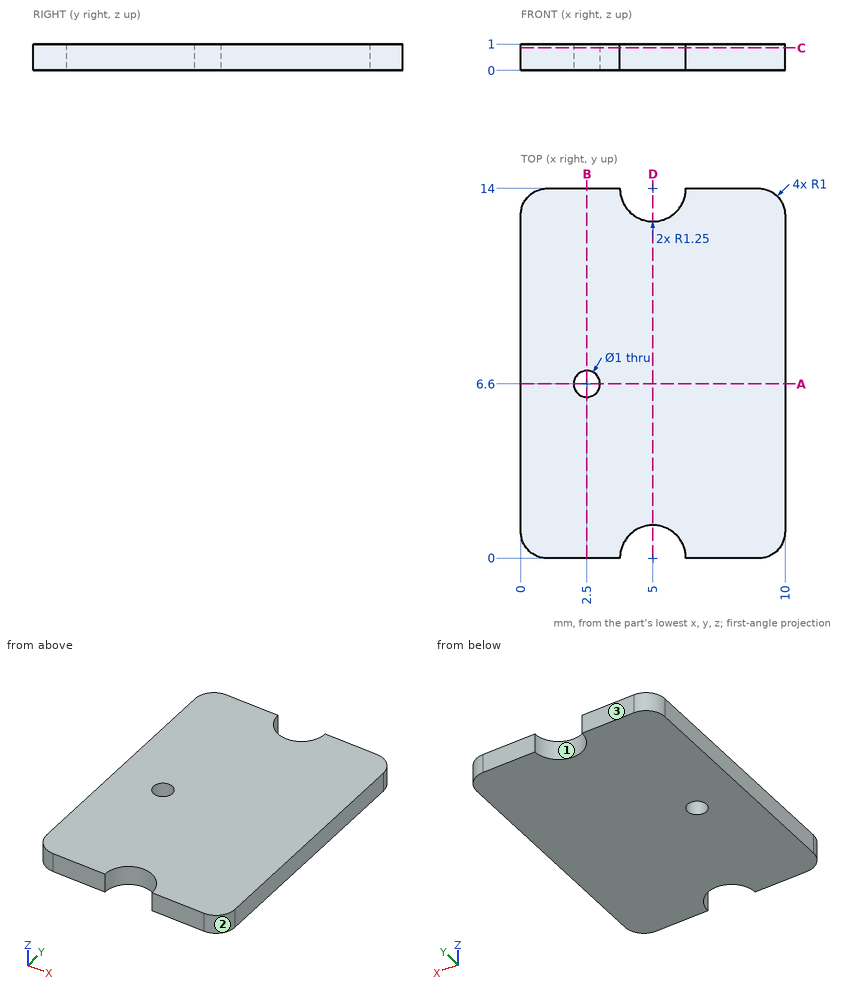
Drawing for the job (mm, zero at the part's lowest x, y, z). Coordinates: 2 decimals unless noted, no trailing zeros. Loops run counter-clockwise (first coordinate to the right, second up) from the corner with the lowest first, then second, coordinate; pieces in that order, holes last. Notation, with made-up numbers: (24, 60.25) - (69, 60.25) arc R17 cw to (69, 83.25) - close; hole circle Ø6 at (-26.75, -8). An arc over 180 degrees is marked (long way). Use CSV: the item, a comma, the result in double quotes. Start each with the question number.
Q1. Cut at B-B, the plane x = 2.5. List the corners of the cut face in (y, z), then the cut area to 3 significant figures.
Q2. Two-plate mould, pull along X, no slides. Class the marked faces 1, 2 and 3: +X half, -X half, draft (parallel to the pull), parting line (faces both ways), or undercut.
Q3. Cut at A-A, the plane y = 6.6. List the corners of the cut face in (x, z).
Q4. Cut at C-C, the plane z = 0.85. List the corners of the cut face in (x, y).
Q5. Probe probe 1 along Y at (x, z) = (2.5, 0.4); probe 2 along X at (y, z) = (7, 0.1); probe 3 along X at (y, z) = (13.75, 0.15). List the from-to ranges inside material, lowest first. Write a range as from..to.
Q6. Cut at D-D, the plane x = 5. List the corners of the cut face in (y, z), then the cut area to 3 significant figures.
Here are the results:
1,outline,"(0, 0) - (6.1, 0) - (6.1, 1) - (0, 1) - close; (7.1, 0) - (14, 0) - (14, 1) - (7.1, 1) - close"
1,area,"13.0 mm2"
2,face 1,"undercut"
2,face 2,"+X half"
2,face 3,"draft"
3,outline,"(0, 0) - (2, 0) - (2, 1) - (0, 1) - close; (3, 0) - (10, 0) - (10, 1) - (3, 1) - close"
4,outline,"(0, 1) arc R1 ccw to (1, 0) - (3.75, 0) arc R1.25 cw to (6.25, 0) - (9, 0) arc R1 ccw to (10, 1) - (10, 13) arc R1 ccw to (9, 14) - (6.25, 14) arc R1.25 cw to (3.75, 14) - (1, 14) arc R1 ccw to (0, 13) - close; hole circle Ø1 at (2.5, 6.6)"
5,probe 1,"0..6.1, 7.1..14"
5,probe 2,"0..2.2, 2.8..10"
5,probe 3,"0.34..3.78, 6.22..9.66"
6,outline,"(1.25, 0) - (12.75, 0) - (12.75, 1) - (1.25, 1) - close"
6,area,"11.5 mm2"
